The model under review builds one solid part; all positions refer to its coordinate system, in mm. A direction names the side the tool comes from. Give positions to 0.01 mm unless a question says otherwise; leave off trailing zeros. Loops run counter-clockwise (first coordinate to the right, second up) from the corner with the lowest first, then second, coordinate; pieces in that order, holes last. Notation, with made-up numbers: (35.5, 81) - (49.5, 81) arc R31 cw to (49.5, 119) - close; hole circle Ø10 at (42.25, 23.5). An arc over 180 degrees is marked (long way). Return JSON: item names as keys, results as strings. Group by question number.
from build123d import *

# Parameters (mm, degrees)
SKETCH1_W           = 10
SKETCH1_H           = 22.5
BOSS_EXTRUDE1_DEPTH = 30
CUT_EXTRUDE1_REACH  = 34.428
SKETCH2_W           = 4
SKETCH2_H           = 17.5
SKETCH3_R           = 0.75
CUT_EXTRUDE2_DEPTH  = 34.564303955
SKETCH4_R           = 0.75
CUT_EXTRUDE3_DEPTH  = 34.564303955


with BuildPart() as part:
    # Sketch1 → Boss-Extrude1 (new body)
    with BuildSketch(Plane.XY):
        Rectangle(SKETCH1_W, SKETCH1_H)
    extrude(amount=BOSS_EXTRUDE1_DEPTH)

    # Sketch2 → Cut-Extrude1 (cut, up to next)
    with BuildSketch(Plane.XY.offset(30), mode=Mode.PRIVATE) as cut_extrude1_sk1:
        with Locations((-2, -2.5)):
            Rectangle(SKETCH2_W, SKETCH2_H)
    cut_extrude1_tool1 = extrude(cut_extrude1_sk1.sketch, amount=-CUT_EXTRUDE1_REACH, mode=Mode.PRIVATE) & part.part
    cut_extrude1 = cut_extrude1_tool1.solids().sort_by_distance((-2, -2.5, 30))[0]
    add(cut_extrude1, mode=Mode.SUBTRACT)

    # Mirror1: Cut-Extrude1 across plane
    add(cut_extrude1.mirror(Plane(origin=(0, 0, 0), x_dir=(0, 0, 1), z_dir=(1, 0, 0))), mode=Mode.SUBTRACT)

    # Sketch3 → Cut-Extrude2 (cut, through all)
    with BuildSketch(Plane(origin=(5, 0, 0), x_dir=(0, 0, -1), z_dir=(1, 0, 0))):
        with Locations((-5.75, -8.75)):
            Circle(SKETCH3_R)
        with Locations((-5.75, 0.5)):
            Circle(SKETCH3_R)
    cut_extrude2 = extrude(amount=-CUT_EXTRUDE2_DEPTH, mode=Mode.SUBTRACT)

    # Mirror2: Cut-Extrude2 across plane
    add(cut_extrude2.mirror(Plane.XY.offset(15)), mode=Mode.SUBTRACT)

    # Sketch4 → Cut-Extrude3 (cut, through all)
    with BuildSketch(Plane.ZY.offset(5)):
        with Locations((15, 0.5)):
            Circle(SKETCH4_R)
    extrude(amount=-CUT_EXTRUDE3_DEPTH, mode=Mode.SUBTRACT)


solid = part.part
Item 1: For P1, Ø1.4, axis at y = -8.75, z = 24.25, coming from the -X side; P2, Ø2.5, axis at x = 0, z = 9, coming from the -Y side, all flat-tipped, find the tip position at first contact; note any pin that passes through.
Item 2: Take a section at D-D (z = 24.25). State the section outline as (x, y) points, then the cut area to 3 significant figures.
Item 3: For L1, parallel to Y at x = 4.65, z = 24.25; L2, parallel to X at y = 4.25, z = 13; L3, parallel to Y at x = 1.25, z = 11, list the stretches that pass through material, from the lowest coordinate up. Write a range as from..to.
Item 4: Mouldability with a two-part tool opening along Y and no side actions: class faces 3 (the face through (0, 6.25, 15)), 4 (the face through (0, 11.25, 15)), 5 (the face through (-4.51, 0.53, 14.25)) as +Y half, -Y half, draft (parallel to the pull), parting line (faces both ways), or undercut.
Item 5: Take a section at C-C (z = 15). State the section outline as (x, y) points, then the cut area to 3 significant figures.
Item 6: Take a section at B-B (y = -8.75). State the section outline as (x, z) points, then the cut area to 3 significant figures.
Item 7: Take a section at A-A (y = 0.5). State how many separate pieces and enclosed holes the cut face has, then the cut area to 3 significant figures.
Item 8: Tool access review of faces 1 (the face through (-4.49, -8.24, 6.3)), 2 (the face through (4, -3, 15)): name each direction out of +Z, -Z, +X, -X, +Y, -Y from which nothing blocks a thin tool from reaching the whole face with its end or side.
Check sheet entries:
{
 "1": {"P1": "passes through", "P2": "stops at y = 6.25"},
 "2": {"outline": "(-5, -11.25) - (-4, -11.25) - (-4, -9.5) - (-5, -9.5) - close; (-5, -8) - (-4, -8) - (-4, -0.25) - (-5, -0.25) - close; (-5, 1.25) - (-4, 1.25) - (-4, 6.25) - (4, 6.25) - (4, 1.25) - (5, 1.25) - (5, 11.25) - (-5, 11.25) - close; (4, -11.25) - (5, -11.25) - (5, -9.5) - (4, -9.5) - close; (4, -8) - (5, -8) - (5, -0.25) - (4, -0.25) - close", "area": "79.0 mm^2"},
 "3": {"L1": "y = -11.25..-9.5, -8..-0.25, 1.25..11.25", "L2": "x = -5..-4, 4..5", "L3": "y = 6.25..11.25"},
 "4": {"face 3": "-Y half", "face 4": "+Y half", "face 5": "undercut"},
 "5": {"outline": "(-5, -11.25) - (-4, -11.25) - (-4, -0.25) - (-5, -0.25) - close; (-5, 1.25) - (-4, 1.25) - (-4, 6.25) - (4, 6.25) - (4, 1.25) - (5, 1.25) - (5, 11.25) - (-5, 11.25) - close; (4, -11.25) - (5, -11.25) - (5, -0.25) - (4, -0.25) - close", "area": "82.0 mm^2"},
 "6": {"outline": "(-5, 0) - (-4, 0) - (-4, 5) - (-5, 5) - close; (-5, 6.5) - (-4, 6.5) - (-4, 23.5) - (-5, 23.5) - close; (-5, 25) - (-4, 25) - (-4, 30) - (-5, 30) - close; (4, 0) - (5, 0) - (5, 5) - (4, 5) - close; (4, 6.5) - (5, 6.5) - (5, 23.5) - (4, 23.5) - close; (4, 25) - (5, 25) - (5, 30) - (4, 30) - close", "area": "54.0 mm^2"},
 "7": {"separate pieces": "8", "enclosed holes": "0", "area": "51.0 mm^2"},
 "8": {"face 1": "+X, -X", "face 2": "+Z, -Z, -Y"}
}
